```python
from build123d import *

# Parameters (mm, degrees)
BASE_FLANGE1_DEPTH           = 214
EDGE_FLANGE1_STRIP_W         = 12
EDGE_FLANGE1_STRIP_H         = 2
EDGE_FLANGE1_STRIP_CUT_DEPTH = 428
EDGE_FLANGE1_DEPTH           = 428
EDGE_FLANGE2_STRIP_W         = 12
EDGE_FLANGE2_STRIP_H         = 2
EDGE_FLANGE2_STRIP_CUT_DEPTH = 428
EDGE_FLANGE2_DEPTH           = 428
SKETCH6_R                    = 2
CUT_EXTRUDE2_DEPTH           = 10
LPATTERN3_COUNT              = 3
LPATTERN3_PITCH              = 174


# Sheet-metal steps are written as plain solids
with BuildPart() as part:
    # Sketch2 → Base-Flange1 (new, symmetric)
    with BuildSketch(Plane.XY):
        with BuildLine():
            Line((-30, 54), (-30, 4))
            ThreePointArc((-30, 4), (-28.828427125, 1.171572875), (-26, 0))
            Line((-26, 0), (0, 0))
            Line((0, 0), (0, 2))
            Line((0, 2), (-26, 2))
            ThreePointArc((-26, 2), (-27.414213562, 2.585786438), (-28, 4))
            Line((-28, 4), (-28, 54))
            Line((-28, 54), (-30, 54))
        make_face()
    extrude(amount=BASE_FLANGE1_DEPTH, both=True)

    # Edge-Flange1 strip (across the edge) → Edge-Flange1 strip cut (cut)
    with BuildSketch(Plane(origin=(-28, 54, -214), x_dir=(0, -1, 0), z_dir=(0, 0, 1))):
        with Locations((-2, -1)):
            Rectangle(EDGE_FLANGE1_STRIP_W, EDGE_FLANGE1_STRIP_H)
    extrude(amount=EDGE_FLANGE1_STRIP_CUT_DEPTH, mode=Mode.SUBTRACT)

    # Edge-Flange1 section (across the edge) → Edge-Flange1 (add)
    with BuildSketch(Plane(origin=(-28, 54, -214), x_dir=(0, -1, 0), z_dir=(0, 0, 1))):
        with BuildLine():
            Line((0, 2), (0, 26))
            Line((0, 26), (2, 26))
            Line((2, 26), (2, 2))
            ThreePointArc((2, 2), (2.585786438, 0.585786438), (4, 0))
            Line((4, 0), (4, -2))
            ThreePointArc((4, -2), (1.171572875, -0.828427125), (0, 2))
        make_face()
    extrude(amount=EDGE_FLANGE1_DEPTH)

    # Edge-Flange2 strip (across the edge) → Edge-Flange2 strip cut (cut)
    with BuildSketch(Plane(origin=(-2, 54, 214), x_dir=(-1, 0, 0), z_dir=(0, 0, -1))):
        with Locations((-2, -1)):
            Rectangle(EDGE_FLANGE2_STRIP_W, EDGE_FLANGE2_STRIP_H)
    extrude(amount=EDGE_FLANGE2_STRIP_CUT_DEPTH, mode=Mode.SUBTRACT)

    # Edge-Flange2 section (across the edge) → Edge-Flange2 (add)
    with BuildSketch(Plane(origin=(-2, 54, 214), x_dir=(-1, 0, 0), z_dir=(0, 0, -1))):
        with BuildLine():
            Line((0, 2), (0, 18))
            Line((0, 18), (2, 18))
            Line((2, 18), (2, 2))
            ThreePointArc((2, 2), (2.585786438, 0.585786438), (4, 0))
            Line((4, 0), (4, -2))
            ThreePointArc((4, -2), (1.171572875, -0.828427125), (0, 2))
        make_face()
    extrude(amount=EDGE_FLANGE2_DEPTH)

    # Sketch6 → Cut-Extrude2 (cut)
    with BuildSketch(Plane(origin=(-28, 0, 0), x_dir=(0, 0, -1), z_dir=(1, 0, 0))):
        with Locations((174, 25)):
            Circle(SKETCH6_R)
    cut_extrude2 = extrude(amount=-CUT_EXTRUDE2_DEPTH, mode=Mode.SUBTRACT)

    # LPattern3: Cut-Extrude2 ×3
    with Locations(*[(0, 0, i * LPATTERN3_PITCH) for i in range(1, LPATTERN3_COUNT)]):
        add(cut_extrude2, mode=Mode.SUBTRACT)


solid = part.part
```
Can you work these out from the model? Positions are in its coordinate system, mm. A direction names the side the tool comes from. Round coordinates to 2 decimals unless told otherwise and drop trailing zeros. Loops run counter-clockwise (first coordinate to the right, second up) from the corner with the lowest first, then second, coordinate; pieces in that order, holes last. Notation, with made-up numbers: M 34,-8 L 60,-8 A38 cw 60,30 Z; hole C 83,-34 d4. An arc over 180 degrees is marked long. Answer in a Markdown table with one row per item.
1. If we section it at B-B, the plane z = -181.5: Please give me the cut outline in (x, y), plus the area to 3 significant figures.
Established:
| item | result |
|---|---|
| outline | M -30,4 A4 ccw -26,0 L 0,0 L 0,2 L -26,2 A2 cw -28,4 L -28,50 A2 cw -26,52 L -6,52 A4 ccw -2,56 L -2,72 L -4,72 L -4,56 A2 cw -6,54 L -26,54 A4 ccw -30,50 Z |
| area | 244 mm² |
2. If we section it at A-A, the plane x = -12.5: Please give me the cut outline in (y, z).
Established:
| item | result |
|---|---|
| outline | M 0,-214 L 2,-214 L 2,214 L 0,214 Z; M 52,-214 L 54,-214 L 54,214 L 52,214 Z |
3. Please list where these lines run through material, in increasing order: line 1 (Y direction, x = -22.25, z = 60.5); line 2 (X direction, y = 9, z = 153); line 3 (Y direction, x = -29.05, z = 0). Write a range as from..to.
Established:
| item | result |
|---|---|
| line 1 | 0..2, 52..54 |
| line 2 | -30..-28 |
| line 3 | 1.41..23, 27..52.59 |
4. On a 3-axis mill with a long thin cutter (end or side, diameter ignored), from which of +Z, -Z, +X, -X, +Y, -Y can I reach the whole of each face in a straight line? I mean faces 5 (the face through (-2, 64, 3)), 6 (the face through (-16, 52, -3)), 7 (the face through (-4, 64, 3)), 8 (the face through (-30, 27, 3)), 9 (the face through (-28.4, 30.8, -214)). Say none if no direction works.
Established:
| item | result |
|---|---|
| face 5 | +Z, -Z, +X, +Y |
| face 6 | +Z, -Z, +X |
| face 7 | +Z, -Z, -X, +Y |
| face 8 | +Z, -Z, -X, +Y, -Y |
| face 9 | -Z, +X, -X, +Y, -Y |
5. If we section it at C-C, the plane y = 11.5: Please give me the cut outline in (x, z).
Established:
| item | result |
|---|---|
| outline | M -30,-214 L -28,-214 L -28,214 L -30,214 Z |
6. Thinking about a two-plate mould opening in Y: for faces 1 (the face through (-28.4, 30.8, 214)), 2 (the face through (-16, 54, -3)), 3 (the face through (-13, 2, 3)), 4 (the face through (-13, 0, 3)), which applies, pulls with the +Y half, pulls with the -Y half, needs draft (parallel to the pull), parting line crosses it, or undercut?
Established:
| item | result |
|---|---|
| face 1 | needs draft |
| face 2 | pulls with the +Y half |
| face 3 | undercut |
| face 4 | pulls with the -Y half |
7. I'm going to push flat-ended pins straight in: pin 1 Ø12 at (y, z) = (47, -36) entering from +X; pin 2 Ø4 at (y, z) = (60.5, 40) entering from -X; pin 3 Ø4.5 at (y, z) = (25, 174) entering from +X; pin 4 Ø2.5 at (y, z) = (25, -174) entering from -X. Where does each tip first touch, or does it pass through?
Established:
| item | result |
|---|---|
| pin 1 | x = -3.35 |
| pin 2 | x = -4 |
| pin 3 | x = -28 |
| pin 4 | through |
